Can you work these out from the model? Positions are in its coordinate system, mm. A direction names the side the tool comes from. Give positions to 0.01 mm unless a question says otherwise; leave off trailing zeros. Order: outer loops, then holes, each group sorted by start corner. A loop starts at its lowest first (then second) coordinate and runs counter-clockwise, first axis right, second up. Notation, with made-up numbers: M -25,-10.5 L 14,-10.5 A14 ccw 14,10.5 Z; hole C 28.5,19 d4. An arc over 180 degrees is marked long. Use one line per item in the form item = value. Start each with the question number.
1. I need wall thicknesses on L1, parallel to Y at x = 80, z = 2.25; L2, parallel to X at y = 30, z = 4.25; L3, parallel to Y at x = 82.5, z = 3.25. Which ranges of each line are inside material? Lowest first, please.
2. I want a section at C-C, the plane x = 71. List the corners of the cut face in (y, z) for me, and give its area (3 significant figures).
3. For faces 5 (the face through (5.43, 37.65, 4.07)), 6 (the face through (154.573, 64.784, 5.115)), 7 (the face through (30.79, 60.45, 4.06)), which set-ups out of +Z, -Z, +X, -X, +Y, -Y let a thin tool reach every point of the face, with its end or its side?
4. Will these pins go through, and if not, where does the flat tip stop? P1, Ø6, axis at x = 51, y = 62.5, coming from the -Z side; P2, Ø3, axis at y = 6, z = 4, coming from the +X side; P3, Ø2.5, axis at y = 6, z = 4, coming from the -X side; P4, Ø20, axis at x = 80, y = 20, coming from the +Z side.
5. We'd pull the mould along Z, two halves only. Please class faces 1 (the face through (12, 6, 4)), 2 (the face through (79, 37, 0)), 3 (the face through (154.57, 4.35, 4.07)), 4 (the face through (30.08, 12.394, 4.056)): +Z half, -Z half, draft (parallel to the pull), parting line (faces both ways), or undercut.
6. I want a section at A-A, the plane y = 52. List the corners of the cut face in (x, z) for me.
7. I want a section at B-B, the plane x = 120. List the corners of the cut face in (y, z) for me, and give its area (3 significant figures).
```python
from build123d import *

# Parameters (mm, degrees)
BOX_W          = 160
BOX_H          = 72
BOX_DEPTH      = 8
SKETCH_R       = 1.65
HOLE_DEPTH     = 11.00858
HOLE_TIPS_R    = 1.65
SKETCH001_R    = 1.65
HOLE001_DEPTH  = 11.00858
HOLE001_TIPS_R = 1.65
SKETCH002_R    = 12.5
HOLE002_DEPTH  = 8.001


with BuildPart() as part:
    # Box → Box (new body)
    with BuildSketch(Plane.XY):
        with Locations((80, 36)):
            Rectangle(BOX_W, BOX_H)
    extrude(amount=BOX_DEPTH)

    # Sketch (on Face1 of BaseFeature) → Hole (cut)
    with BuildSketch(Plane(origin=(0, 0, 0), x_dir=(0, -1, 0), z_dir=(-1, 0, 0))):
        with Locations((-66, 4)):
            Circle(SKETCH_R)
        with Locations((-36, 4)):
            Circle(SKETCH_R)
        with Locations((-6, 4)):
            Circle(SKETCH_R)
    extrude(amount=-HOLE_DEPTH, mode=Mode.SUBTRACT)

    # Hole tips → Hole tip 1 section 0
    with BuildSketch(Plane(origin=(11.00858, 0, 0), x_dir=(0, -1, 0), z_dir=(-1, 0, 0)), mode=Mode.PRIVATE) as hole_tip_1_s0:
        with Locations((-66, 4)):
            Circle(HOLE_TIPS_R)
    loft([hole_tip_1_s0.sketch, Vertex(12, 66, 4)], mode=Mode.SUBTRACT)

    # Hole tips → Hole tip 2 section 0
    with BuildSketch(Plane(origin=(11.00858, 0, 0), x_dir=(0, -1, 0), z_dir=(-1, 0, 0)), mode=Mode.PRIVATE) as hole_tip_2_s0:
        with Locations((-36, 4)):
            Circle(HOLE_TIPS_R)
    loft([hole_tip_2_s0.sketch, Vertex(12, 36, 4)], mode=Mode.SUBTRACT)

    # Hole tips → Hole tip 3 section 0
    with BuildSketch(Plane(origin=(11.00858, 0, 0), x_dir=(0, -1, 0), z_dir=(-1, 0, 0)), mode=Mode.PRIVATE) as hole_tip_3_s0:
        with Locations((-6, 4)):
            Circle(HOLE_TIPS_R)
    loft([hole_tip_3_s0.sketch, Vertex(12, 6, 4)], mode=Mode.SUBTRACT)

    # Sketch001 (on Face9 of Hole) → Hole001 (cut)
    with BuildSketch(Plane.YZ.offset(160)):
        with Locations((6, 4)):
            Circle(SKETCH001_R)
        with Locations((36, 4)):
            Circle(SKETCH001_R)
        with Locations((66, 4)):
            Circle(SKETCH001_R)
    extrude(amount=-HOLE001_DEPTH, mode=Mode.SUBTRACT)

    # Hole001 tips → Hole001 tip 1 section 0
    with BuildSketch(Plane.YZ.offset(148.99142), mode=Mode.PRIVATE) as hole001_tip_1_s0:
        with Locations((6, 4)):
            Circle(HOLE001_TIPS_R)
    loft([hole001_tip_1_s0.sketch, Vertex(148, 6, 4)], mode=Mode.SUBTRACT)

    # Hole001 tips → Hole001 tip 2 section 0
    with BuildSketch(Plane.YZ.offset(148.99142), mode=Mode.PRIVATE) as hole001_tip_2_s0:
        with Locations((36, 4)):
            Circle(HOLE001_TIPS_R)
    loft([hole001_tip_2_s0.sketch, Vertex(148, 36, 4)], mode=Mode.SUBTRACT)

    # Hole001 tips → Hole001 tip 3 section 0
    with BuildSketch(Plane.YZ.offset(148.99142), mode=Mode.PRIVATE) as hole001_tip_3_s0:
        with Locations((66, 4)):
            Circle(HOLE001_TIPS_R)
    loft([hole001_tip_3_s0.sketch, Vertex(148, 66, 4)], mode=Mode.SUBTRACT)

    # Sketch002 (on Face3 of Hole001) → Hole002 (cut, through all)
    with BuildSketch(Plane.XY.offset(8)):
        with Locations((40, 52)):
            Circle(SKETCH002_R)
        with Locations((40, 20)):
            Circle(SKETCH002_R)
        with Locations((120, 52)):
            Circle(SKETCH002_R)
        with Locations((120, 20)):
            Circle(SKETCH002_R)
        with Locations((80, 52)):
            Circle(SKETCH002_R)
        with Locations((80, 20)):
            Circle(SKETCH002_R)
    extrude(amount=-HOLE002_DEPTH, mode=Mode.SUBTRACT)


solid = part.part
```
Check result:
q1.L1 = 0 to 7.5, 32.5 to 39.5, 64.5 to 72
q1.L2 = 0 to 32.5, 47.5 to 72.5, 87.5 to 112.5, 127.5 to 160
q1.L3 = 0 to 7.75, 32.25 to 39.75, 64.25 to 72
q2.outline = M 0,0 L 11.33,0 L 11.33,8 L 0,8 Z; M 28.67,0 L 43.33,0 L 43.33,8 L 28.67,8 Z; M 60.67,0 L 72,0 L 72,8 L 60.67,8 Z
q2.area = 298 mm2
q3.face_5 = -X
q3.face_6 = +X
q3.face_7 = +Z, -Z
q4.P1 = 0
q4.P2 = 148.9
q4.P3 = 11.25
q4.P4 = through
q5.face_1 = undercut
q5.face_2 = -Z half
q5.face_3 = undercut
q5.face_4 = draft
q6.outline = M 0,0 L 27.5,0 L 27.5,8 L 0,8 Z; M 52.5,0 L 67.5,0 L 67.5,8 L 52.5,8 Z; M 92.5,0 L 107.5,0 L 107.5,8 L 92.5,8 Z; M 132.5,0 L 160,0 L 160,8 L 132.5,8 Z
q7.outline = M 0,0 L 7.5,0 L 7.5,8 L 0,8 Z; M 32.5,0 L 39.5,0 L 39.5,8 L 32.5,8 Z; M 64.5,0 L 72,0 L 72,8 L 64.5,8 Z
q7.area = 176 mm2
